Input: part model. Units: mm. Frame: model coordinates. Face numbers are marked on the shaded views. Give positions to 0.01 mm unless a question says otherwise; leave off trailing zeros. Loops run counter-clockwise (first coordinate to the right, second up) from the corner with the lowest first, then second, coordinate; pieces in that order, holes last. Notation, with made-up numbers: M -19.75,22 L -7.75,22 A21 ccw -7.75,47 Z; hole C 11.5,58 d7. An arc over 180 degrees is marked long. Use CSV: the item, a comma, the result in double quotes. Start each with the question number.
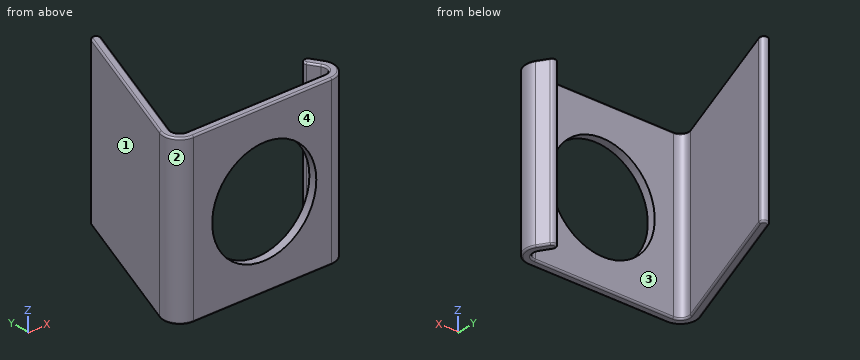
from build123d import *

# Parameters (mm, degrees)
PAD_DEPTH    = 20
FILLET_R     = 0.2
SKETCH001_R  = 6.35529
POCKET_DEPTH = 5


with BuildPart() as part:
    # Sketch → Pad (new body)
    with BuildSketch(Plane.XY):
        with BuildLine():
            Line((13.174844, 20.172385), (6.753583, 2.689539))
            ThreePointArc((6.753583, 2.689539), (6.990976, 0.855246), (8.630958, 0))
            Line((8.630958, 0), (25.485807, 0))
            ThreePointArc((25.485807, 0), (27.23513, 1.030532), (27.18172, 3.060131))
            Line((27.18172, 3.060131), (26.428525, 4.265033))
            ThreePointArc((26.428525, 4.265033), (25.739514, 4.423978), (25.580568, 3.734967))
            Line((25.580568, 3.734967), (26.333764, 2.530066))
            ThreePointArc((25.485807, 1), (26.360469, 1.515266), (26.333764, 2.530066))
            Line((25.485807, 1), (8.630958, 1))
            ThreePointArc((7.69227, 2.34477), (7.810967, 1.427623), (8.630958, 1))
            Line((7.69227, 2.34477), (14.113531, 19.827615))
            ThreePointArc((14.113531, 19.827615), (13.816572, 20.469344), (13.174844, 20.172385))
        make_face()
    extrude(amount=PAD_DEPTH)

    # Fillet
    fillet_edges = [part.edges().sort_by_distance(p)[0] for p in [
        (10.902901, 11.086192, 20),
        (13.816572, 20.469344, 20),
        (9.964213, 11.430962, 20),
        (6.990976, 0.855246, 20),
        (17.058382, 0, 20),
        (27.23513, 1.030532, 20),
        (26.805123, 3.662582, 20),
        (25.739514, 4.423978, 20),
        (25.957166, 3.132516, 20),
        (26.360469, 1.515266, 20),
        (17.058382, 1, 20),
        (7.810967, 1.427623, 20),
        (10.902901, 11.086192, 0),
        (13.816572, 20.469344, 0),
        (9.964213, 11.430962, 0),
        (6.990976, 0.855246, 0),
        (17.058382, 0, 0),
        (27.23513, 1.030532, 0),
        (26.805123, 3.662582, 0),
        (25.739514, 4.423978, 0),
        (25.957166, 3.132516, 0),
        (26.360469, 1.515266, 0),
        (17.058382, 1, 0),
        (7.810967, 1.427623, 0),
    ]]
    fillet(fillet_edges, radius=FILLET_R)

    # Sketch001 (on Face35 of Fillet) → Pocket (cut)
    with BuildSketch(Plane.XZ):
        with Locations((17.266081, 9.78687)):
            Circle(SKETCH001_R)
    extrude(amount=-POCKET_DEPTH, mode=Mode.SUBTRACT)


solid = part.part
Item 1: Section B-B (z = 12.5). Output: boundary loops of the cut face in (x, y).
Item 2: Mould query, pull axis Y, two halves, no side actions, for the marked faces 1, 2, 3 and 4. Classes: +Y half, -Y half, draft (parallel to the pull), parting line (faces both ways), or undercut.
Item 3: Section D-D (x = 19). Output: boundary loops of the cut face in (y, z), then the cut area to 3 significant figures.
Item 4: Section C-C (x = 24.5). Output: boundary loops of the cut face in (y, z).
Item 5: Material intervals for line 1 (Y direction, x = 21.25, z = 4.5); line 2 (X direction, y = 1.75, z = 17.75); line 3 (X direction, y = 4.25, z = 6.5), sorted ascending.
Item 6: Section A-A (x = 16.25). Output: boundary loops of the cut face in (y, z).
Item 7: First-contact query: pin 1 Ø1.5 at (y, z) = (14, 2.5) entering from -X; pin 2 Ø8 at (y, z) = (15.5, 3) entering from +X; pin 3 Ø3 at (x, z) = (18.5, 3) entering from +Y. Flat tips, straight axial feed; report the tip coordinate or a pass-through.
Recorded:
1,outline,"M 6.75,2.69 A2 ccw 8.63,0 L 11.52,0 L 11.52,1 L 8.63,1 A1 cw 7.69,2.34 L 14.11,19.83 A0.5 ccw 13.17,20.17 Z; M 23.01,0 L 25.49,0 A2 ccw 27.18,3.06 L 26.43,4.27 A0.5 ccw 25.58,3.73 L 26.33,2.53 A1 cw 25.49,1 L 23.01,1 Z"
2,face 1,"+Y half"
2,face 2,"parting line"
2,face 3,"undercut"
2,face 4,"-Y half"
3,outline,"M 0,0.2 A0.2 ccw 0.2,0 L 0.8,0 A0.2 ccw 1,0.2 L 1,3.67 L 0,3.67 Z; M 0,15.9 L 1,15.9 L 1,19.8 A0.2 ccw 0.8,20 L 0.2,20 A0.2 ccw 0,19.8 Z"
3,area,"7.74 mm²"
4,outline,"M 0,0.2 A0.2 ccw 0.2,0 L 0.8,0 A0.2 ccw 1,0.2 L 1,19.8 A0.2 ccw 0.8,20 L 0.2,20 A0.2 ccw 0,19.8 Z"
5,line 1,"0 to 1"
5,line 2,"6.65 to 7.66, 26.45 to 27.47"
5,line 3,"7.33 to 8.39, 25.57 to 26.44"
6,outline,"M 0,0.2 A0.2 ccw 0.2,0 L 0.8,0 A0.2 ccw 1,0.2 L 1,3.51 L 0,3.51 Z; M 0,16.06 L 1,16.06 L 1,19.8 A0.2 ccw 0.8,20 L 0.2,20 A0.2 ccw 0,19.8 Z"
7,pin 1,"x = 10.63"
7,pin 2,"x = 13.99"
7,pin 3,"y = 1"
